Work out the finished part from the listing and answer in its coordinate system (mm). Round coordinates to 2 decimals unless told otherwise and drop trailing zeros. Write each loop counter-clockwise with the first axis right and the second up, starting at its lowest first coordinate (ties: lowest second). Pieces come first, ordered by that corner, then holes. Notation, with made-up numbers: M 76.5,-0.75 L 107.5,-0.75 A21 ccw 107.5,11.25 Z; hole C 87.5,35 d2. An arc over 180 degrees is marked long. Answer in a Markdown table with one row per item.
```python
from build123d import *

# Parameters (mm, degrees)
SKETCH1_W                        = 1223.9625
SKETCH1_H                        = 1976.755
BOSS_EXTRUDE1_DEPTH              = 3.175
CUT_EXTRUDE1_DEPTH               = 1163.519443002
F_1_4_CLEARANCE_HOLE1_D          = 6.7564
F_27_64_0_42188_DIAMETER_HOLE1_D = 10.715752
F_27_64_0_42188_DIAMETER_HOLE3_D = 10.715752
F_27_64_0_42188_DIAMETER_HOLE2_D = 10.715752
SKETCH9_W                        = 1223.9625
SKETCH9_H                        = 9.525
CUT_EXTRUDE2_DEPTH               = 1163.519443002
FILLET1_R                        = 6.35
FILLET2_R                        = 6.35
F_27_64_0_42188_DIAMETER_HOLE4_D = 10.715752
CUT_EXTRUDE3_DEPTH               = 1155.432150283


with BuildPart() as part:
    # Sketch1 → Boss-Extrude1 (new, symmetric)
    with BuildSketch(Plane.XY):
        Rectangle(SKETCH1_W, SKETCH1_H)
    extrude(amount=BOSS_EXTRUDE1_DEPTH, both=True)

    # Sketch2 → Cut-Extrude1 (cut, through all)
    with BuildSketch(Plane.XY.offset(3.175)):
        Polygon((294.48125, 313.3725), (611.98125, 313.3725), (611.98125, -23.1775), (611.98125, -988.3775), (-611.98125, -988.3775), (-611.98125, -23.1775), (294.48125, -23.1775), align=None)
    extrude(amount=-CUT_EXTRUDE1_DEPTH, mode=Mode.SUBTRACT)

    # 1/4 Clearance Hole1 (through all)
    with Locations(Plane.XY.offset(3.175)):
        with Locations((-542.13125, -0.9525), (-288.13125, -0.9525), (-59.53125, -0.9525), (194.46875, -0.9525)):
            Hole(F_1_4_CLEARANCE_HOLE1_D / 2)

    # 27/64 (0.42188) Diameter Hole1 (through all)
    with Locations(Plane(origin=(573.88125, 516.5725, 3.175), x_dir=(1, 0, 0), z_dir=(0, 0, 1))):
        with Locations((0, 0), (-1154.1125, 0)):
            Hole(F_27_64_0_42188_DIAMETER_HOLE1_D / 2)

    # 27/64 (0.42188) Diameter Hole3 (through all)
    with Locations(Plane(origin=(275.43125, 327.66, 3.175), x_dir=(1, 0, 0), z_dir=(0, 0, 1))):
        with Locations((0, 0), (304.8, 0), (304.8, 19.05), (0, 19.05)):
            Hole(F_27_64_0_42188_DIAMETER_HOLE3_D / 2)

    # 27/64 (0.42188) Diameter Hole2 (through all)
    with Locations(Plane.XY.offset(3.175)):
        with Locations((205.58125, 924.8775), (573.88125, 940.7525), (0, 940.7525), (-580.23125, 940.7525), (-205.58125, 924.8775)):
            Hole(F_27_64_0_42188_DIAMETER_HOLE2_D / 2)

    # Sketch9 → Cut-Extrude2 (cut, through all)
    with BuildSketch(Plane.XY.offset(3.175)):
        with Locations((0, 983.615)):
            Rectangle(SKETCH9_W, SKETCH9_H)
    extrude(amount=-CUT_EXTRUDE2_DEPTH, mode=Mode.SUBTRACT)

    # Fillet1
    fillet1_edges = [part.edges().sort_by_distance(p)[0] for p in [
        (294.48125, 313.3725, 0),
    ]]
    fillet(fillet1_edges, radius=FILLET1_R)

    # Fillet2
    fillet2_edges = [part.edges().sort_by_distance(p)[0] for p in [
        (611.98125, 978.8525, 0),
        (-611.98125, 978.8525, 0),
        (294.48125, -23.1775, 0),
        (611.98125, 313.3725, 0),
        (-611.98125, -23.1775, 0),
    ]]
    fillet(fillet2_edges, radius=FILLET2_R)

    # 27/64 (0.42188) Diameter Hole4 (through all)
    with Locations(Plane.XY.offset(3.175)):
        with Locations((-573.88125, 782.0025), (-548.48125, 782.0025)):
            Hole(F_27_64_0_42188_DIAMETER_HOLE4_D / 2)

    # Sketch12 → Cut-Extrude3 (cut, through all)
    with BuildSketch(Plane.XY.offset(3.175)):
        with BuildLine():
            Line((288.13125, -16.8275), (-592.93125, -16.8275))
            ThreePointArc((-592.93125, -16.8275), (-597.421378061, -14.967628061), (-599.28125, -10.4775))
            Line((-599.28125, -10.4775), (-599.28125, 972.5025))
            ThreePointArc((-599.28125, 972.5025), (-597.421378061, 976.992628061), (-592.93125, 978.8525))
            Line((-592.93125, 978.8525), (-605.63125, 978.8525))
            ThreePointArc((-605.63125, 978.8525), (-610.121378061, 976.992628061), (-611.98125, 972.5025))
            Line((-611.98125, 972.5025), (-611.98125, -16.8275))
            ThreePointArc((-611.98125, -16.8275), (-610.121378061, -21.317628061), (-605.63125, -23.1775))
            Line((-605.63125, -23.1775), (288.13125, -23.1775))
            ThreePointArc((288.13125, -23.1775), (292.621378061, -21.317628061), (294.48125, -16.8275))
            Line((294.48125, -16.8275), (294.48125, -10.4775))
            ThreePointArc((294.48125, -10.4775), (292.621378061, -14.967628061), (288.13125, -16.8275))
        make_face()
    extrude(amount=-CUT_EXTRUDE3_DEPTH, mode=Mode.SUBTRACT)


solid = part.part
```
1. The part is cut by section B-B (y = 205). Determine the outline of the cut face in (x, z) (3 decimals), plus the area to 3 significant figures.
Calculated:
| item | result |
|---|---|
| outline | M -599.281,-3.175 L 294.481,-3.175 L 294.481,3.175 L -599.281,3.175 Z |
| area | 5,680 mm² |
2. The part is cut by section A-A (z = -2). Count the separate pieces of the cut face and the enclosed holes in it, plus the area to 3 significant figures.
Calculated:
| item | result |
|---|---|
| separate pieces | 1 |
| enclosed holes | 17 |
| area | 1,100,000 mm² |
3. Given pin 1 (12.5 mm diameter, centred on x = 573.88, y = 516.57, fed in from +Z) (3 decimals); pin 2 (1.9 mm diameter, centred on x = 527, z = -0.5, fed in from -Y), each flat-ended and moving along its own axis, determine where each tip first touches the part or whether it passes through.
Calculated:
| item | result |
|---|---|
| pin 1 | stops at z = 3.175 |
| pin 2 | stops at y = 313.37 |
4. Consider line 1 along Y through (x, z) = (0, 0); line 2 along Y through (x, z) = (338.5, -1); line 3 along X through (y, z) = (256.5, -1.5). Determine where each line is inside the solid, lowest interval first. Write a range as from..to.
Calculated:
| item | result |
|---|---|
| line 1 | y = -16.83..935.39, 946.11..978.85 |
| line 2 | y = 313.37..978.85 |
| line 3 | x = -599.28..294.48 |
